Drawing for the job (mm, zero at the part's lowest x, y, z). Round coordinates to 2 decimals unless told otherwise and drop trailing zeros. Loops run counter-clockwise (first coordinate to the right, second up) from the corner with the lowest first, then second, coordinate; pieces in that order, holes last. Notation, with made-up numbers: (68.5, 70.5) -> (100.5, 70.5) arc R22 ccw to (100.5, 93.5) -> close; hole circle Ø3 at (3, 30). An arc over 180 degrees is marked (long way). Put each result on its own line as item: value. Start each with the question number.
Item 1: Cut at D-D, the plane z = 0.3. Count the separate pieces of the cut face and the enclosed holes in it.
Item 2: Drill centre lines: probe 1 along Y at (x, z) = (7.5, 0.2); probe 2 along X at (y, z) = (2.5, 0.3) (1 decimal); probe 3 along Y at (x, z) = (1.5, 0.35). Where is each one in solid material? Low to high. Write a range as [from, to].
Item 3: Cut at A-A, the plane y = 1.5. List the corners of the cut face in (x, z).
Item 4: Cut at C-C, the plane y = 7.5. List the corners of the cut face in (x, z).
Item 5: Pull direction Z, two halves, no side cores. Call the marked faces 1 and 2: +Z half, -Z half, draft (parallel to the pull), parting line (faces both ways), or undercut.
Item 6: Flat gauge pin, fed straight in: pin 1 Ø1.8 at (x, y) = (3.26, 11.74) entering from +Z. Where does the tip first touch, or does it go through?
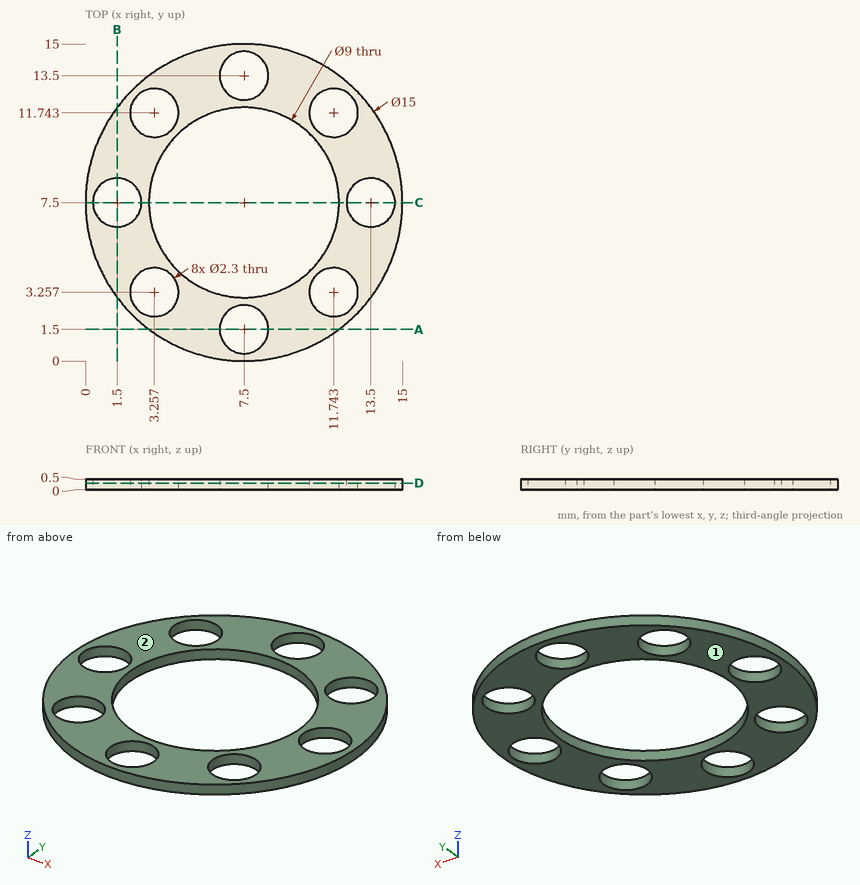
Reply:
1. separate pieces: 1
1. enclosed holes: 9
2. probe 1: y = [0, 0.35], [2.65, 3], [12, 12.35], [14.65, 15]
2. probe 2: x = [1.9, 2.4], [4.1, 6.9], [8.1, 10.9], [12.6, 13.1]
2. probe 3: y = [3, 6.35], [8.65, 12]
3. outline: (3, 0) -> (6.35, 0) -> (6.35, 0.5) -> (3, 0.5) -> close; (8.65, 0) -> (12, 0) -> (12, 0.5) -> (8.65, 0.5) -> close
4. outline: (0, 0) -> (0.35, 0) -> (0.35, 0.5) -> (0, 0.5) -> close; (2.65, 0) -> (3, 0) -> (3, 0.5) -> (2.65, 0.5) -> close; (12, 0) -> (12.35, 0) -> (12.35, 0.5) -> (12, 0.5) -> close; (14.65, 0) -> (15, 0) -> (15, 0.5) -> (14.65, 0.5) -> close
5. face 1: -Z half
5. face 2: +Z half
6. pin 1: passes through
